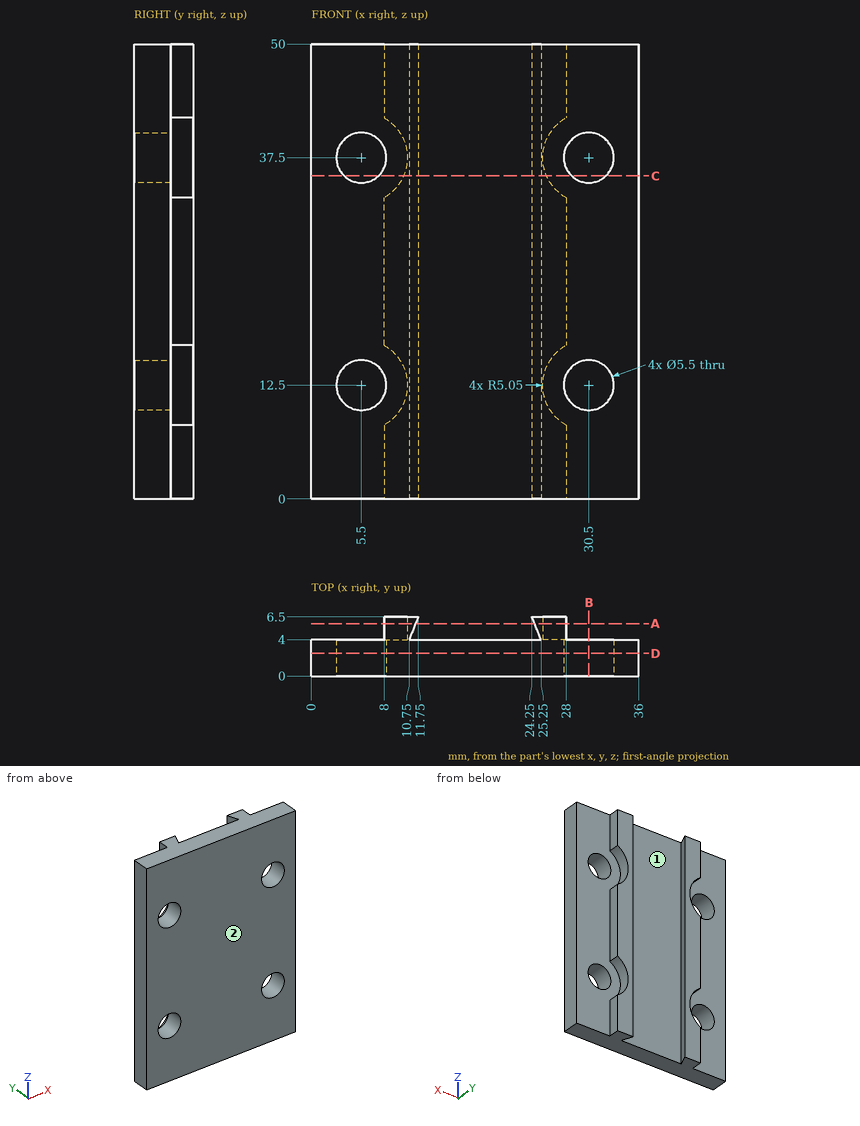
Source: three-view drawing plus pictorial views. Frame: mm from the lowest corner of the part. Coordinates: 2 decimals unless noted, no trailing zeros. Order: outer loops, then holes, each group sorted by start corner. A loop starts at its lowest first (then second) coordinate and runs counter-clockwise, first axis right, second up.
1) Ray query, probe 1 along Z at (x, y) = (30.5, 1.9); probe 2 along X at (y, z) = (2.5, 12.5); probe 3 along Y at (x, z) = (12, 38.5). Return the intervals inside material, ascending.
Result sheet:
probe 1: z = 0 to 9.75, 15.25 to 34.75, 40.25 to 50
probe 2: x = 0 to 2.75, 8.25 to 27.75, 33.25 to 36
probe 3: y = 0 to 4
2) First-contact query: P1, Ø2, axis at y = 5.5, z = 44, coming from the +X side; P2, Ø4.5, axis at x = 15.5, z = 27.5, coming from the +Y side; P3, Ø0.8, axis at y = 5.5, z = 5, coming from the -X side. Flat tips, straight axial feed; report the tip coordinate or a pass-through.
Result sheet:
P1: stops at x = 28
P2: stops at y = 4
P3: stops at x = 8
3) Section C-C (z = 35.5). Return loops of the section in (x, y), then the cut area to 3 significant figures.
Result sheet:
outline: (0, 0) - (3.61, 0) - (3.61, 4) - (0, 4) - close; (7.39, 0) - (28.61, 0) - (28.61, 4) - (25.86, 4) - (25.86, 6.5) - (24.25, 6.5) - (25.25, 4) - (10.75, 4) - (11.75, 6.5) - (10.14, 6.5) - (10.14, 4) - (7.39, 4) - close; (32.39, 0) - (36, 0) - (36, 4) - (32.39, 4) - close
area: 119 mm2
4) Section D-D (y = 2.5). Return loops of the section in (x, z).
Result sheet:
outline: (0, 0) - (36, 0) - (36, 50) - (0, 50) - close; hole circle Ø5.5 at (5.5, 12.5); hole circle Ø5.5 at (5.5, 37.5); hole circle Ø5.5 at (30.5, 12.5); hole circle Ø5.5 at (30.5, 37.5)
5) Draft query along X for the marked faces 1 and 2. Return one class per face: released by +X, released by -X, zero draft, split by the parting line, or undercut.
Result sheet:
face 1: undercut
face 2: zero draft
6) Section B-B (x = 30.5). Return loops of the section in (y, z).
Result sheet:
outline: (0, 0) - (4, 0) - (4, 9.75) - (0, 9.75) - close; (0, 15.25) - (4, 15.25) - (4, 34.75) - (0, 34.75) - close; (0, 40.25) - (4, 40.25) - (4, 50) - (0, 50) - close
7) Section A-A (y = 5.75). Return loops of the section in (x, z).
Result sheet:
outline: (8, 0) - (11.45, 0) - (11.45, 50) - (8, 50) - (8, 41.89) arc R5.05 cw to (8, 33.11) - (8, 16.89) arc R5.05 cw to (8, 8.11) - close; (24.55, 0) - (28, 0) - (28, 8.11) arc R5.05 cw to (28, 16.89) - (28, 33.11) arc R5.05 cw to (28, 41.89) - (28, 50) - (24.55, 50) - close
